```python
from build123d import *

# Parameters (mm, degrees)
SKETCH1_R               = 19.304
SKETCH1_R_2             = 15.24
BOSS_EXTRUDE1_DEPTH     = 12.7
SKETCH2_W               = 25.4
SKETCH2_H               = 38.923585408
BOSS_EXTRUDE2_DEPTH     = 0.4064
CUT_EXTRUDE1_DEPTH      = 56.997301217
CUT_EXTRUDE1_DEPTH_BACK = 56.997301217
SKETCH3_R               = 2.4892
FILLET1_R               = 7.46


with BuildPart() as part:
    # Sketch1 → Boss-Extrude1 (new, symmetric)
    with BuildSketch(Plane(origin=(0, 0, 0), x_dir=(0, 0, -1), z_dir=(1, 0, 0))):
        Circle(SKETCH1_R)
        Circle(SKETCH1_R_2, mode=Mode.SUBTRACT)
    extrude(amount=BOSS_EXTRUDE1_DEPTH, both=True)

    # Sketch2 → Boss-Extrude2 (add)
    with BuildSketch(Plane(origin=(0, -19.304, 0), x_dir=(1, 0, 0), z_dir=(0, 1, 0))):
        with Locations((0, -19.461792704)):
            Rectangle(SKETCH2_W, SKETCH2_H)
    extrude(amount=BOSS_EXTRUDE2_DEPTH)

    # Sketch3 → Cut-Extrude1 (cut, two sides: drawn at the far end of the back side and taken through both)
    with BuildSketch(Plane(origin=(0, -18.8976, 0), x_dir=(1, 0, 0), z_dir=(0, 1, 0)).offset(-CUT_EXTRUDE1_DEPTH_BACK)):
        with Locations(Location((0, -30.211385408, 0), (0, 0, 270))):
            Circle(SKETCH3_R)
    extrude(amount=CUT_EXTRUDE1_DEPTH + CUT_EXTRUDE1_DEPTH_BACK, mode=Mode.SUBTRACT)

    # Fillet1
    fillet1_edges = [part.edges().sort_by_distance(p)[0] for p in [
        (12.7, -19.1008, 38.923585408),
        (-12.7, -19.1008, 38.923585408),
    ]]
    fillet(fillet1_edges, radius=FILLET1_R)


solid = part.part
```
For this review, take the finished solid that the model builds, in its own axes (mm). Round coordinates to 2 decimals unless told otherwise and drop trailing zeros. Loops run counter-clockwise (first coordinate to the right, second up) from the corner with the lowest first, then second, coordinate; pieces in that order, holes last.
Q1. To check wall thickness, follow line 1 along Y through (x, z) = (0, 0); line 2 along Z through (x, y) = (-9.5, -0.5); line 3 along Y through (x, z) = (-11.25, 9). State the ranges of each line that lie inside material, in increasing order.
Result sheet:
line 1: y = -19.3 to -15.24, 15.24 to 19.3
line 2: z = -19.3 to -15.23, 15.23 to 19.3
line 3: y = -19.3 to -18.9, -17.08 to -12.3, 12.3 to 17.08
Q2. Add section A-A on x = 0. Write out the cut boundary in (y, z).
Result sheet:
outline: (-19.3, 0) arc R19.3 ccw (long way) to (-18.9, 3.94) - (-18.9, 27.72) - (-19.3, 27.72) - close; (-19.3, 32.7) - (-18.9, 32.7) - (-18.9, 38.92) - (-19.3, 38.92) - close; hole circle Ø30.48 at (0, 0)
Q3. Add section D-D on x = -4.5. Write out the cut boundary in (y, z).
Result sheet:
outline: (-19.3, 0) arc R19.3 ccw (long way) to (-18.9, 3.94) - (-18.9, 38.92) - (-19.3, 38.92) - close; hole circle Ø30.48 at (0, 0)
Q4. Insertion check: pin 1 Ø5.5 at (x, z) = (0, 30.21) entering from +Y; pin 2 Ø12.5 at (x, z) = (1.5, 14) entering from +Y; pin 3 Ø5 at (x, y) = (-2.5, -1) entering from +Z. Each pin has a flat end and moves straight along its axis. Give the tip position at first contact, or say it passes through.
Result sheet:
pin 1: stops at y = -18.9
pin 2: stops at y = 17.68
pin 3: stops at z = 19.3
Q5. Add section C-C on z = 18.5. Write out the cut boundary in (x, y), plus the area to 3 significant figures.
Result sheet:
outline: (-12.7, -19.3) - (12.7, -19.3) - (12.7, -18.9) - (-12.7, -18.9) - close; (-12.7, -5.51) - (12.7, -5.51) - (12.7, 5.51) - (-12.7, 5.51) - close
area: 290 mm2
Q6. Mouldability with a two-part tool opening along Y and no side actions: class faces 1 (the face through (-0.18, -14.88, 3.3)), 2 (the face through (0.7, -19.1, 32.6)), 3 (the face through (0, -19.304, 19)) as +Y half, -Y half, draft (parallel to the pull), parting line (faces both ways), or undercut.
Result sheet:
face 1: undercut
face 2: draft
face 3: -Y half
Q7. Add section B-B on y = 0. Write out the cut boundary in (x, z).
Result sheet:
outline: (-12.7, -19.3) - (12.7, -19.3) - (12.7, -15.24) - (-12.7, -15.24) - close; (-12.7, 15.24) - (12.7, 15.24) - (12.7, 19.3) - (-12.7, 19.3) - close
